from build123d import *

# Parameters (mm, degrees)
SKETCH_W              = 80
SKETCH_H              = 20
PAD_DEPTH             = 52.5
SKETCH001_R           = 2.75
POCKET_DEPTH          = 20.001
SKETCH002_R           = 4.75
POCKET001_DEPTH       = 5.54
SKETCH003_W           = 21
SKETCH003_H           = 45
POCKET002_DEPTH       = 20.001
FILLET_R              = 5
CLONE_PLACEMENT_ANGLE = 90


with BuildPart() as part:
    # Sketch → Pad (new body, symmetric)
    with BuildSketch(Plane.XZ):
        with Locations((0, -10)):
            Rectangle(SKETCH_W, SKETCH_H)
    extrude(amount=PAD_DEPTH, both=True)

    # Sketch001 (on Face4 of Pad) → Pocket (cut, through all)
    with BuildSketch(Plane(origin=(0, 0, 0), x_dir=(-1, 0, 0), z_dir=(0, 0, 1))):
        with Locations((-30, -42.5)):
            Circle(SKETCH001_R)
        with Locations((30, -42.5)):
            Circle(SKETCH001_R)
        with Locations((-10, 42.5)):
            Circle(SKETCH001_R)
        with Locations((10, 42.5)):
            Circle(SKETCH001_R)
        with Locations((-10, 22.5)):
            Circle(SKETCH001_R)
        with Locations((10, 22.5)):
            Circle(SKETCH001_R)
        with Locations((-10, -42.5)):
            Circle(SKETCH001_R)
        with Locations((10, -42.5)):
            Circle(SKETCH001_R)
    extrude(amount=-POCKET_DEPTH, mode=Mode.SUBTRACT)

    # Sketch002 (on Face2 of Pocket) → Pocket001 (cut)
    with BuildSketch(Plane(origin=(0, 0, 0), x_dir=(-1, 0, 0), z_dir=(0, 0, 1))):
        with Locations((-10, 42.5)):
            Circle(SKETCH002_R)
        with Locations((10, 42.5)):
            Circle(SKETCH002_R)
        with Locations((-10, 22.5)):
            Circle(SKETCH002_R)
        with Locations((10, 22.5)):
            Circle(SKETCH002_R)
        with Locations((10, -42.5)):
            Circle(SKETCH002_R)
        with Locations((30, -42.5)):
            Circle(SKETCH002_R)
        with Locations((-30, -42.5)):
            Circle(SKETCH002_R)
        with Locations((-10, -42.5)):
            Circle(SKETCH002_R)
    extrude(amount=-POCKET001_DEPTH, mode=Mode.SUBTRACT)

    # Sketch003 (on Face2 of Pocket001) → Pocket002 (cut, through all)
    with BuildSketch(Plane(origin=(0, 0, 0), x_dir=(-1, 0, 0), z_dir=(0, 0, 1))):
        with Locations((-29.5, 30)):
            Rectangle(SKETCH003_W, SKETCH003_H)
        with Locations((29.5, 30)):
            Rectangle(SKETCH003_W, SKETCH003_H)
    extrude(amount=-POCKET002_DEPTH, mode=Mode.SUBTRACT)

    # Fillet
    fillet_edges = [part.edges().sort_by_distance(p)[0] for p in [
        (40, -7.5, -10),
        (19, -7.5, -10),
        (19, -52.5, -10),
        (-19, -52.5, -10),
        (-19, -7.5, -10),
        (-40, -7.5, -10),
    ]]
    fillet(fillet_edges, radius=FILLET_R)


with BuildPart() as part_1:
    # Clone placement: moved
    add(part.part.moved(Location((-52.5, 40, 0))).rotate(Axis((-52.5, 40, 0), (0, 0, -1)), CLONE_PLACEMENT_ANGLE))


solid = part_1.part
For this review, take the finished solid that the model builds, in its own axes (mm). A direction names the side the tool comes from. Give positions to 0.01 mm unless a question says otherwise; leave off trailing zeros. Loops run counter-clockwise (first coordinate to the right, second up) from the corner with the lowest first, then second, coordinate; pieces in that order, holes last. Notation, with made-up numbers: M -0.75,19.5 L 55.25,19.5 A26 ccw 55.25,55.5 Z; hole C -11.75,-4 d10. An arc over 180 degrees is marked long. Put each result on its own line as item: value. Start each with the question number.
(1) Wall thickness on L1, parallel to Y at x = -10, z = -1.85; L2, parallel to Y at x = -95, z = -2.05; L3, parallel to X at y = 30, z = -9.5: over which ranges is each line inside the solid? List them lowest first.
(2) The part is to be moulded in two halves that separate along X. For faces 3 (the flat face through (-82, 21, -10)), 4 (the flat face through (-60, 10, -10)), 5 (the flat face through (-7, 70, -5.54)), say which applies: +X half, -X half, draft (parallel to the pull), parting line (faces both ways), or undercut.
(3) Add section C-C, the plane z = -10.75. Give the number of separate pieces and of enclosed holes in the cut face, then the cut area to 3 significant figures.
(4) Add section B-B, the plane x = -75. Write out the cut boundary in (y, z), then the cut area to 3 significant figures.
(5) Add section A-A, the plane y = 50. Write out the cut boundary in (x, z), then the cut area to 3 significant figures.
(6) For pin 1 (5 mm diameter, centred on x = -75, y = 31, fed in from +Z); pin 2 (1.5 mm diameter, centred on y = 64.5, z = -6.5, fed in from -X); pin 3 (1.5 mm diameter, centred on x = -58, z = -4.5, fed in from +Y), all flat-tipped, find the tip position at first contact; note any pin that passes through.
(7) Machinability: for faces 1 (the cylindrical face through (-58, 79, -10)), 2 (the cylindrical face through (-7.11, 66.23, -2.73)), which of the approach directions +Z, -Z, +X, -X, +Y, -Y give a long, thin tool a straight path to every point of the face, cutting with its end or side? Answer none if there is none.
Result:
1. L1: y = 0 to 5.25, 14.75 to 25.25, 34.75 to 45.25, 54.75 to 65.25, 74.75 to 80
1. L2: y = 21 to 25.25, 34.75 to 45.25, 54.75 to 59
1. L3: x = -105 to -97.75, -92.25 to -77.75, -72.25 to -12.75, -7.25 to 0
2. face 3: draft
2. face 4: -X half
2. face 5: undercut
3. separate pieces: 1
3. enclosed holes: 8
3. area: 6,310 mm^2
4. outline: M 21,-20 L 27.25,-20 L 27.25,-5.54 L 25.25,-5.54 L 25.25,0 L 21,0 Z; M 32.75,-20 L 47.25,-20 L 47.25,-5.54 L 45.25,-5.54 L 45.25,0 L 34.75,0 L 34.75,-5.54 L 32.75,-5.54 Z; M 52.75,-20 L 59,-20 L 59,0 L 54.75,0 L 54.75,-5.54 L 52.75,-5.54 Z
4. area: 496 mm^2
5. outline: M -105,-20 L -97.75,-20 L -97.75,-5.54 L -99.75,-5.54 L -99.75,0 L -105,0 Z; M -92.25,-20 L -77.75,-20 L -77.75,-5.54 L -79.75,-5.54 L -79.75,0 L -90.25,0 L -90.25,-5.54 L -92.25,-5.54 Z; M -72.25,-20 L -12.75,-20 L -12.75,-5.54 L -14.75,-5.54 L -14.75,0 L -70.25,0 L -70.25,-5.54 L -72.25,-5.54 Z; M -7.25,-20 L 0,-20 L 0,0 L -5.25,0 L -5.25,-5.54 L -7.25,-5.54 Z
5. area: 1,700 mm^2
6. pin 1: stops at z = -5.54
6. pin 2: stops at x = -60.01
6. pin 3: stops at y = 79.47
7. face 1: +Z, -Z, -X, +Y
7. face 2: +Z
